Geometry: final body of the model. Coordinates: model frame, mm. A direction names the side the tool comes from. Round coordinates to 2 decimals unless told otherwise and drop trailing zeros. Order: outer loops, then holes, each group sorted by start corner. A loop starts at its lowest first (then second) coordinate and runs counter-clockwise, first axis right, second up. Notation, with made-up numbers: M 70,78 L 78,78 A26 ccw 78,104 Z; hole C 70.25,-6 d2. An arc over 180 degrees is marked long. Put each result on its own line as item: value. Start each with the question number.
1) Section A-A, the plane x = 0. Return loops of the section in (y, z), then the cut area to 3 significant figures.
2) Draft query along Y for faces 1 (the flat face through (50, 98, -30)), 2 (the flat face through (-1, 95, -28)), 3 (the cylindrical face through (17.805, 96.487, -30.028)). Return one class per face: pulls with the +Y half, pulls with the -Y half, needs draft (parallel to the pull), parting line crosses it, or undercut.
3) Access query for faces 4 (the cylindrical face through (41.67, 92.48, -31.01)), 5 (the flat face through (-40, 88, -30)). Directions: +Z, -Z, +X, -X, +Y, -Y. A direction counts if a zero-diameter tool reaches every point of the face in a straight line with its end or side. Return the directions, or none.
4) Section C-C, the plane z = -31.05. Return loops of the section in (x, y).
5) Section D-D, the plane x = -42. Return loops of the section in (y, z), then the cut area to 3 significant figures.
6) Material intervals for probe 1 along X at (y, z) = (95, -30.2); probe 2 along X at (y, z) = (90, -31.1); probe 3 along Y at (x, z) = (18, -28.85), sorted ascending. Write a range as [from, to].
7) Section B-B, the plane x = -18. Return loops of the section in (y, z).
8) First-contact query: P1, Ø6, axis at x = 42, y = 90, coming from the +Z side; P2, Ø5, axis at x = 18, y = 95, coming from the +Z side. Flat tips, straight axial feed; report the tip coordinate or a pass-through.
from build123d import *

# Parameters (mm, degrees)
CYLINDER1716_R     = 2.5
CYLINDER1716_DEPTH = 20
CYLINDER1717_R     = 2.5
CYLINDER1717_DEPTH = 20
CYLINDER1715_R     = 5
CYLINDER1715_DEPTH = 5
CYLINDER1718_R     = 5
CYLINDER1718_DEPTH = 5
CYLINDER1711_R     = 1.5
CYLINDER1711_DEPTH = 60
CYLINDER1712_R     = 1.5
CYLINDER1712_DEPTH = 60
CYLINDER1713_R     = 1.5
CYLINDER1713_DEPTH = 60
CYLINDER1714_R     = 1.5
CYLINDER1714_DEPTH = 60
CYLINDER1701_R     = 3
CYLINDER1701_DEPTH = 48
BOX659_W           = 104
BOX659_H           = 20
BOX659_DEPTH       = 4
CHAMFER057_SIZE    = 4
CHAMFER058_SIZE    = 2


with BuildPart() as obj1:
    # Cylinder1716 → Cylinder1716 (new body)
    with BuildSketch(Plane(origin=(-42, 90, -59), x_dir=(1, 0, 0), z_dir=(0, 0, 1))):
        Circle(CYLINDER1716_R)
    extrude(amount=CYLINDER1716_DEPTH)


with BuildPart() as compound845:
    # Cylinder1717 → Cylinder1717 (new body)
    with BuildSketch(Plane(origin=(42, 90, -59), x_dir=(1, 0, 0), z_dir=(0, 0, 1))):
        Circle(CYLINDER1717_R)
    extrude(amount=CYLINDER1717_DEPTH)

    # Compound845: union obj1
    add(obj1.part)


with BuildPart() as compound845_1:
    # Compound845 placement: moved
    add(compound845.part.moved(Location((0, 0, 18))))


with BuildPart() as obj2:
    # Cylinder1715 → Cylinder1715 (new body)
    with BuildSketch(Plane(origin=(-42, 90, -59), x_dir=(1, 0, 0), z_dir=(0, 0, 1))):
        Circle(CYLINDER1715_R)
    extrude(amount=CYLINDER1715_DEPTH)


with BuildPart() as compound844:
    # Cylinder1718 → Cylinder1718 (new body)
    with BuildSketch(Plane(origin=(42, 90, -59), x_dir=(1, 0, 0), z_dir=(0, 0, 1))):
        Circle(CYLINDER1718_R)
    extrude(amount=CYLINDER1718_DEPTH)

    # Compound844: union obj2
    add(obj2.part)


with BuildPart() as compound844_1:
    # Compound844 placement: moved
    add(compound844.part.moved(Location((0, 0, 29))))


with BuildPart() as obj3:
    # Cylinder1711 → Cylinder1711 (new body)
    with BuildSketch(Plane(origin=(18, 85, -57), x_dir=(1, 0, 0), z_dir=(0, 0, 1))):
        Circle(CYLINDER1711_R)
    extrude(amount=CYLINDER1711_DEPTH)


with BuildPart() as obj4:
    # Cylinder1712 → Cylinder1712 (new body)
    with BuildSketch(Plane(origin=(-18, 85, -57), x_dir=(1, 0, 0), z_dir=(0, 0, 1))):
        Circle(CYLINDER1712_R)
    extrude(amount=CYLINDER1712_DEPTH)


with BuildPart() as obj5:
    # Cylinder1713 → Cylinder1713 (new body)
    with BuildSketch(Plane(origin=(-18, 95, -57), x_dir=(1, 0, 0), z_dir=(0, 0, 1))):
        Circle(CYLINDER1713_R)
    extrude(amount=CYLINDER1713_DEPTH)


with BuildPart() as compound847:
    # Cylinder1714 → Cylinder1714 (new body)
    with BuildSketch(Plane(origin=(18, 95, -57), x_dir=(1, 0, 0), z_dir=(0, 0, 1))):
        Circle(CYLINDER1714_R)
    extrude(amount=CYLINDER1714_DEPTH)

    # Compound847: union obj3, obj4, obj5
    add(obj3.part)
    add(obj4.part)
    add(obj5.part)


with BuildPart() as obj6:
    # Cylinder1701 → Cylinder1701 (new body)
    with BuildSketch(Plane(origin=(0, 90, -55), x_dir=(1, 0, 0), z_dir=(0, 0, 1))):
        Circle(CYLINDER1701_R)
    extrude(amount=CYLINDER1701_DEPTH)


with BuildPart() as chamfer058:
    # Box659 → Box659 (new body)
    with BuildSketch(Plane(origin=(-52, 80, -32), x_dir=(1, 0, 0), z_dir=(0, 0, 1))):
        with Locations((52, 10)):
            Rectangle(BOX659_W, BOX659_H)
    extrude(amount=BOX659_DEPTH)

    # Cut345: cut obj6
    add(obj6.part, mode=Mode.SUBTRACT)

    # Cut351: cut Compound847
    add(compound847.part, mode=Mode.SUBTRACT)

    # Cut353: cut Compound844
    add(compound844_1.part, mode=Mode.SUBTRACT)

    # Cut350: cut Compound845
    add(compound845_1.part, mode=Mode.SUBTRACT)

    # Chamfer057
    chamfer057_edges = [chamfer058.edges().sort_by_distance(p)[0] for p in [
        (-52, 100, -30),
        (52, 100, -30),
    ]]
    chamfer(chamfer057_edges, length=CHAMFER057_SIZE)

    # Chamfer058
    chamfer058_edges = [chamfer058.edges().sort_by_distance(p)[0] for p in [
        (-52, 88, -28),
        (52, 88, -28),
    ]]
    chamfer(chamfer058_edges, length=CHAMFER058_SIZE)


solid = chamfer058.part
Result sheet:
1. outline: M 80,-32 L 87,-32 L 87,-28 L 80,-28 Z; M 93,-32 L 100,-32 L 100,-28 L 93,-28 Z
1. area: 56.0 mm2
2. face 1: pulls with the +Y half
2. face 2: needs draft
2. face 3: undercut
3. face 4: +Z, -Z
3. face 5: +Z
4. outline: M -52,80 L 52,80 L 52,96 L 48,100 L -48,100 L -52,96 Z; hole C -42,90 d5; hole C -18,85 d3; hole C -18,95 d3; hole C 0,90 d6; hole C 18,85 d3; hole C 18,95 d3; hole C 42,90 d5
5. outline: M 80,-32 L 87.5,-32 L 87.5,-30 L 85,-30 L 85,-28 L 80,-28 Z; M 92.5,-32 L 100,-32 L 100,-28 L 95,-28 L 95,-30 L 92.5,-30 Z
5. area: 50.0 mm2
6. probe 1: x = [-52, -19.5], [-16.5, 16.5], [19.5, 52]
6. probe 2: x = [-52, -44.5], [-39.5, -3], [3, 39.5], [44.5, 52]
6. probe 3: y = [80, 83.5], [86.5, 93.5], [96.5, 100]
7. outline: M 80,-32 L 83.5,-32 L 83.5,-28 L 80,-28 Z; M 86.5,-32 L 93.5,-32 L 93.5,-28 L 86.5,-28 Z; M 96.5,-32 L 100,-32 L 100,-28 L 96.5,-28 Z
8. P1: stops at z = -30
8. P2: stops at z = -28
